```python
from build123d import *

# Parameters (mm, degrees)
SKETCH_7_R      = 15
EXTRUDE_2_DEPTH = 12
FILLET_1_R      = 0.5


with BuildPart() as part:
    # Sketch 7 → Extrude 2 (new body)
    with BuildSketch(Plane(origin=(0, 0, 0), x_dir=(0, 0, -1), z_dir=(1, 0, 0))):
        with BuildLine():
            Line((18.114916731, -13.345403397), (16.503520778, -12.415063509))
            Line((16.503520778, -12.415063509), (19.003520778, -8.084936491))
            Line((19.003520778, -8.084936491), (20.614916731, -9.015276378))
            ThreePointArc((20.614916731, -9.015276378), (19.485571585, 11.25), (2.5, 22.360679775))
            Line((2.5, 22.360679775), (2.5, 20.5))
            Line((2.5, 20.5), (-2.5, 20.5))
            Line((-2.5, 20.5), (-2.5, 22.360679775))
            ThreePointArc((-2.5, 22.360679775), (-19.485571585, 11.25), (-20.614916731, -9.015276378))
            Line((-20.614916731, -9.015276378), (-19.003520778, -8.084936491))
            Line((-19.003520778, -8.084936491), (-16.503520778, -12.415063509))
            Line((-16.503520778, -12.415063509), (-18.114916731, -13.345403397))
            ThreePointArc((-18.114916731, -13.345403397), (0, -22.5), (18.114916731, -13.345403397))
        make_face()
        Circle(SKETCH_7_R, mode=Mode.SUBTRACT)
    extrude(amount=EXTRUDE_2_DEPTH)

    # Fillet 1
    fillet_1_edges = [part.edges().sort_by_distance(p)[0] for p in [
        (0, -22.5, 0),
        (0, 11.25, 19.485571585),
        (0, 11.25, -19.485571585),
        (12, 11.25, 19.485571585),
        (0, 0, 15),
        (12, 0, 15),
        (12, -22.5, 0),
        (12, 11.25, -19.485571585),
    ]]
    fillet(fillet_1_edges, radius=FILLET_1_R)


solid = part.part
```
Here's how the part is built. I have some questions about the finished solid (model axes, mm). A direction names the side the tool comes from. Round coordinates to 2 decimals unless told otherwise and drop trailing zeros. Order: outer loops, then holes, each group sorted by start corner. A loop starts at its lowest first (then second) coordinate and runs counter-clockwise, first axis right, second up. Notation, with made-up numbers: (18.5, 51) -> (65.5, 51) arc R32 cw to (65.5, 79) -> close; hole circle Ø8 at (6, -9.75). An arc over 180 degrees is marked (long way). Use a Markdown table: item, result. Add a question column.
(1) For pin 1 Ø5.5 at (x, z) = (7, -1) entering from +Y; pin 2 Ø3 at (y, z) = (-7, -10) entering from +X; pin 3 Ø4 at (x, y) = (10.5, 11) entering from -Z; pin 4 Ø3 at (x, y) = (7, 17) entering from -Z, each with a flat end and sliding along its axis, tell me the tip position at first contact or that it passes through.
(2) Suppose I cut it at B-B, the plane z = 0. Please give me the cut outline in (x, y).
(3) I need wall thicknesses on line 1 along Y through (x, z) = (7.25, 0); line 2 along Z through (x, y) = (0.75, -12.5); line 3 along Z through (x, y) = (9.25, -13). Which ranges of each line are inside material? Lowest first, please.
(4) If we mould it in two halves opening along Y, with no side actions, what happens to faces 6 (the face through (0, 15, 5)), 7 (the face through (5.92, -10.22, 17.77)), 8 (the face through (5.923, 10.994, -19.631))? For each: released by +Y, released by -Y, zero draft, split by the parting line, or undercut.
(5) Suppose I cut it at A-A, the plane x = 6.75. Please give me the cut outline in (y, z).
(6) For faces 1 (the face through (6, 21, -2.5)), 2 (the face through (5.916, -10.28, -17.736)), 3 (the face through (5.916, -12.874, 17.298)), 4 (the face through (5.916, -8.544, -19.798)), 5 (the face through (5.916, -12.887, -17.32)), which set-ups out of +Z, -Z, +X, -X, +Y, -Y let a thin tool reach every point of the face, with its end or its side?
Verdict:
| question | item | result |
|---|---|---|
| 1 | pin 1 | y = 22.36 |
| 1 | pin 2 | through |
| 1 | pin 3 | z = -20.62 |
| 1 | pin 4 | z = -16.31 |
| 2 | outline | (0, -22) arc R0.5 ccw to (0.5, -22.5) -> (11.5, -22.5) arc R0.5 ccw to (12, -22) -> (12, -15.5) arc R0.5 ccw to (11.5, -15) -> (0.5, -15) arc R0.5 ccw to (0, -15.5) -> close; (0, 15.5) arc R0.5 ccw to (0.5, 15) -> (11.5, 15) arc R0.5 ccw to (12, 15.5) -> (12, 20.5) -> (0, 20.5) -> close |
| 3 | line 1 | -22.5 to -15, 15 to 20.5 |
| 3 | line 2 | -16.65 to -8.29, 8.29 to 16.65 |
| 3 | line 3 | -17.52 to -7.48, 7.48 to 17.52 |
| 4 | face 6 | zero draft |
| 4 | face 7 | undercut |
| 4 | face 8 | split by the parting line |
| 5 | outline | (-13.35, -18.11) -> (-12.42, -16.5) -> (-8.08, -19) -> (-9.02, -20.61) arc R22.5 ccw to (22.36, -2.5) -> (20.5, -2.5) -> (20.5, 2.5) -> (22.36, 2.5) arc R22.5 ccw to (-9.02, 20.61) -> (-8.08, 19) -> (-12.42, 16.5) -> (-13.35, 18.11) arc R22.5 ccw to start; hole circle Ø30 at (0, 0) |
| 6 | face 1 | +X, -X, +Y |
| 6 | face 2 | +X, -X |
| 6 | face 3 | +Z, +X, -X |
| 6 | face 4 | +X, -X, -Y |
| 6 | face 5 | -Z, +X, -X |
